```python
from build123d import *

# Parameters (mm, degrees)
F0_R     = 10.16
F1_DEPTH = 15.7734
F2_DEPTH = 40.2336
F3_R     = 3.302


with BuildPart() as f1:
    # F0 (on Top) → F1 (new body)
    with BuildSketch(Plane.XY):
        with BuildLine():
            ThreePointArc((5.272246, 28.084409), (21.990737, 18.246591), (28.575, 0))
            ThreePointArc((28.575, 0), (21.990737, -18.246591), (5.272246, -28.084409))
            Line((5.272246, -28.084409), (55.139294, -18.72294))
            ThreePointArc((55.139294, -18.72294), (70.674464, 0), (55.139294, 18.72294))
            Line((55.139294, 18.72294), (5.272246, 28.084409))
        make_face()
        with Locations((53.975, 0)):
            Circle(F0_R, mode=Mode.SUBTRACT)
    extrude(amount=F1_DEPTH)

    # F0 (on Top) → F2 (join)
    with BuildSketch(Plane.XY):
        with BuildLine():
            ThreePointArc((5.272246, -28.084409), (21.990737, -18.246591), (28.575, 0))
            ThreePointArc((28.575, 0), (21.990737, 18.246591), (5.272246, 28.084409))
            ThreePointArc((5.272246, 28.084409), (-28.575, 0), (5.272246, -28.084409))
        make_face()
        with BuildLine():
            ThreePointArc((-13.447765, 4.826), (0, 14.2875), (13.447765, 4.826))
            Line((13.447765, 4.826), (18.5293, 4.826))
            Line((18.5293, 4.826), (18.5293, -4.826))
            Line((18.5293, -4.826), (13.447765, -4.826))
            ThreePointArc((13.447765, -4.826), (0, -14.2875), (-13.447765, -4.826))
            Line((-13.447765, -4.826), (-18.5293, -4.826))
            Line((-18.5293, -4.826), (-18.5293, 4.826))
            Line((-18.5293, 4.826), (-13.447765, 4.826))
        make_face(mode=Mode.SUBTRACT)
        with BuildLine():
            ThreePointArc((-13.447765, -4.826), (-14.2875, 0), (-13.447765, 4.826))
            Line((-13.447765, 4.826), (-18.5293, 4.826))
            Line((-18.5293, 4.826), (-18.5293, -4.826))
            Line((-18.5293, -4.826), (-13.447765, -4.826))
        make_face()
    extrude(amount=F2_DEPTH)

    # F3
    f3_edges = [f1.edges().sort_by_distance(p)[0] for p in [
        (-5.272246, 28.084409, 40.2336),
    ]]
    fillet(f3_edges, radius=F3_R)


solid = f1.part
```
Design review of the part built by this model. Coordinates are the model's own, in mm. A direction names the side the tool comes from. Give positions to 0.01 mm unless a question says otherwise; leave off trailing zeros. Write each question's results on one line, items separated by ' | '. Start each with the question number.
Q1. For pin 1 (1.5 mm diameter, centred on x = -10.5, z = 9.5, fed in from -Y); pin 2 (4 mm diameter, centred on y = -5, z = 29, fed in from -X); pin 3 (12 mm diameter, centred on x = 53.975, y = 0, fed in from -Z); pin 4 (10 mm diameter, centred on x = -8, z = 23.5, fed in from -Y), all flat-tipped, find the tip position at first contact; note any pin that passes through.
Q2. Mouldability with a two-part tool opening along X and no side actions: class faces 1 (the cylindrical face through (70.67, -0.37, 7.78)), 2 (the flat face through (20, 0, 0)), 3 (the flat face through (16, -4.826, 20)) as +X half, -X half, draft (parallel to the pull), parting line (faces both ways), or undercut.
Q3. Add section B-B on z = 10.5. State how many separate pieces and enclosed holes the cut face has, and give its area (3 significant figures).
Q4. Wall thickness on L1, parallel to X at y = 1.5, z = 7; L2, parallel to Y at x = 0.5, z = 34; L3, parallel to Z at x = 41, y = 0: over which ranges is each line inside the solid? List them lowest first. Write a range as from..to.
Q5. Machinability: for faces 4 (the flat face through (18.529, 0, 20)), 5 (the flat face through (11, -11, 40.234)), which of the approach directions +Z, -Z, +X, -X, +Y, -Y give a long, thin tool a straight path to every point of the face, cutting with its end or side? Answer none if there is none.
Found:
1) pin 1: stops at y = -26.86 | pin 2: stops at x = -28.42 | pin 3: passes through | pin 4: stops at y = -28.42
2) face 1: +X half | face 2: draft | face 3: undercut
3) separate pieces: 1 | enclosed holes: 2 | area: 3,340 mm2
4) L1: x = -28.54..-14.21, 18.53..43.93, 64.02..70.62 | L2: y = -28.57..-14.28, 14.28..28.57 | L3: z = 0..15.77
5) face 4: +Z, -Z | face 5: +Z, +X, -X, +Y, -Y
